Geometry check sheet. Reference: the model listing, model coordinates, mm. Give positions to 0.01 mm unless a question says otherwise; leave off trailing zeros. Loops run counter-clockwise (first coordinate to the right, second up) from the corner with the lowest first, then second, coordinate; pieces in that order, holes last.
Autodesk Inventor part; units mm, degrees
ref_plane "YZ Plane" through (0, 0, 0) normal (1, 0, 0) x (0, 1, 0)
ref_plane "XZ Plane" through (0, 0, 0) normal (0, 1, 0) x (-1, 0, 0)
ref_plane "XY Plane" through (0, 0, 0) normal (0, 0, 1) x (1, 0, 0)
sketch "Sketch1" plane through (0, 0, 0) normal (0, 1, 0) x (-1, 0, 0)
  arc A0 (34.7717, -25.2969) -> (36.6925, 22.4201) centre (0, 0) ccw
  circle A1 centre (28.6854, -13.0153) radius 1.5
  circle A2 centre (29.0479, 12.1849) radius 1.5
  line L0 (33.6483, 20.8328) -> (30.9628, 19.4812)
  arc A3 (32.7365, 13.7321) -> (30.5518, 18.0787) centre (0, 0) ccw
  arc A4 (37.3473, 15.6662) -> (34.9611, 20.4443) centre (0, 0) ccw
  arc A5 (34.9611, 20.4443) -> (33.6483, 20.8328) centre (34.0979, 19.9395) ccw
  arc A6 (30.9628, 19.4812) -> (30.5518, 18.0787) centre (31.4124, 18.5879) ccw
  line L1 (34.5435, 24.12) -> (27.3337, 20.4914)
  arc A7 (34.3646, 21.4319) -> (33.0708, 23.3788) centre (0, 0) ccw
  arc A8 (27.7564, 17.8489) -> (26.9661, 19.0218) centre (0, 0) ccw
  arc A9 (27.3337, 20.4914) -> (26.9661, 19.0218) centre (27.7833, 19.5982) ccw
  arc A10 (36.6925, 22.4201) -> (35.8263, 23.7798) centre (0, 0) ccw
  arc A11 (35.8263, 23.7798) -> (34.5435, 24.12) centre (34.9931, 23.2268) ccw
  circle A12 centre (29.253, -24.2541) radius 1.5
  arc A13 (27.2186, -20.8101) -> (33.1098, -25.315) centre (29.253, -24.2541) ccw
  arc A14 (28.0626, 15.0184) -> (30.379, 9.4963) centre (29.0479, 12.1849) ccw
  arc A15 (28.6009, 16.4618) -> (27.7564, 17.8489) centre (0, 0) ccw
  arc A16 (30.0933, -10.3662) -> (27.619, -15.8194) centre (28.6854, -13.0153) ccw
  arc A17 (31.5176, -9.7795) -> (31.7859, 8.8689) centre (0, 0) ccw
  arc A18 (26.7939, -19.2636) -> (28.1155, -17.2777) centre (0, 0) ccw
  arc A19 (30.0933, -10.3662) -> (31.5176, -9.7795) centre (30.5625, -9.4832) ccw
  arc A20 (28.1155, -17.2777) -> (27.619, -15.8194) centre (27.2635, -16.7541) ccw
  arc A21 (31.7859, 8.8689) -> (30.379, 9.4963) centre (30.8227, 8.6001) ccw
  arc A22 (28.0626, 15.0184) -> (28.6009, 16.4618) centre (27.7342, 15.963) ccw
  arc A23 (33.3556, -25.5029) -> (34.7717, -25.2969) centre (33.963, -24.7086) ccw
  arc A24 (26.7939, -19.2636) -> (26.9984, -20.6418) centre (27.6058, -19.8474) ccw
  arc A25 (34.2723, -21.5792) -> (33.0708, 23.3788) centre (0, 0) ccw
  arc A26 (30.182, -18.6894) -> (30.5518, 18.0787) centre (0, 0) ccw
  line L2 (32.8186, -21.8408) -> (30.4248, -20.0103)
  arc A27 (32.8186, -21.8408) -> (34.2723, -21.5792) centre (33.426, -21.0464) ccw
  arc A28 (30.182, -18.6894) -> (30.4248, -20.0103) centre (31.0322, -19.2159) ccw
  line L3 (33.3556, -25.5029) -> (33.1098, -25.315)
  line L4 (30.1876, -23.0805) -> (30.1642, -23.0625)
  line L5 (27.2186, -20.8101) -> (26.9984, -20.6418)
  point P0 (26.2158, -20.0433)
  point P1 (29.6958, -19.4528)
  dimension "d2" = 3
  dimension "d0" = 1
  dimension "d1" = 8
  dimension "d3" = 3
  dimension "d4" = 43
  dimension "d5" = 33
  dimension "d6" = 33
  dimension "d7" = 2.5339
  dimension "d8" = 3.4819
  dimension "d9" = 29.0479
  dimension "d10" = 1
  dimension "d11" = 1
  dimension "d12" = 40.5
  dimension "d13" = 1
  dimension "d14" = 1
  dimension "d15" = 43
  dimension "d16" = 40.5
  dimension "d17" = 35.5
  dimension "d18" = 64.12
  dimension "d19" = 2.5829
  dimension "d20" = 0.0025
  dimension "d21" = 35.1283
  dimension "d22" = 6.2779
  dimension "d23" = 40.0956
  dimension "d24" = 0.0494
  dimension "d25" = 37.8965
  dimension "d26" = 40.9793
  dimension "d27" = 30.7911
  dimension "d28" = 9.8494
  dimension "d29" = 8.7909
  dimension "d30" = 37.6697
  dimension "d31" = 0.0165
  dimension "d32" = 0
  dimension "d33" = 6.0158
  dimension "d34" = 0.0025
extrude "Extrusion1" add sketch "Sketch1" along normal blind 3
properties part number "Reverse Gear Link 1 updated" material "Copper"
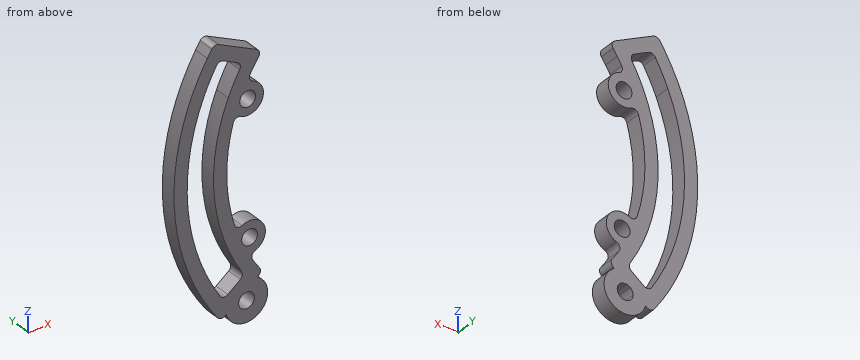
1) Sectioned sample at D-D on y = 1.2. Count the separate pieces of the cut face and the enclosed holes in it, plus the area to 3 significant figures.
2) Sectioned sample at A-A on z = -12. Enter the section's corners in (x, y).
3) Depth check by flat-ended pin: P1, Ø1, axis at y = 0.5, z = -15.5, coming from the +X side. Enter the tip coordinate at first touch or a pass-through.
4) Scan lines: line 1 along X through (y, z) = (1.3, 0); line 2 along Z through (x, y) = (-29.25, 0.6); line 3 along Z through (x, y) = (-30, 1.5). Record each from-to range of solid material in increasing order.
5) Sectioned sample at C-C on x = -38.75. Enter the section's corners in (y, z), plus the area to 3 significant figures.
6) Sectioned sample at B-B on z = -1. Enter the section's corners in (x, y).
Determined:
1. separate pieces: 1
1. enclosed holes: 4
1. area: 331 mm2
2. outline: (-41.29, 0) - (-38.68, 0) - (-38.68, 3) - (-41.29, 3) - close; (-33.41, 0) - (-29.79, 0) - (-29.79, 3) - (-33.41, 3) - close; (-27.58, 0) - (-25.86, 0) - (-25.86, 3) - (-27.58, 3) - close
3. P1: stops at x = -26.44
4. line 1: x = -43 to -40.5, -35.5 to -33
4. line 2: z = -28.25 to -25.75, -22.75 to -14.4, -11.63 to -10.07, 9.19 to 10.7, 13.67 to 21.46
4. line 3: z = -28.18 to -25.55, -22.95 to -13.74, -12.29 to -10.32, 9.34 to 11.03, 13.34 to 21.83
5. outline: (0, -18.64) - (3, -18.64) - (3, -11.78) - (0, -11.78) - close; (0, 11.78) - (3, 11.78) - (3, 18.64) - (0, 18.64) - close
5. area: 41.2 mm2
6. outline: (-42.99, 0) - (-40.49, 0) - (-40.49, 3) - (-42.99, 3) - close; (-35.49, 0) - (-32.98, 0) - (-32.98, 3) - (-35.49, 3) - close
